Can you work these out from the drawing? Everything is in mm from the part's minimum corner. A direction names the side the tool comes from. Coordinates: 2 decimals unless noted, no trailing zeros. Order: outer loops, then holes, each group sorted by start corner. A loop starts at its lowest first (then second) coordinate and runs counter-clockwise, first axis right, second up. Notation, with made-up numbers: (18, 27.5) -> (49, 27.5) arc R4 ccw to (49, 32.5) -> close; hole circle Ø7 at (32.25, 32). An arc over 180 degrees is marked (long way). Return JSON: item names as keys, results as strings. Group by question number.
1) If I drill on probe 1 along Y at (x, z) = (9.5, 11); probe 2 along Z at (x, y) = (10, 6), over which ranges is the centre line in solid material (lowest first)? Write a range as from..to.
2) If we section it at B-B, the plane x = 5.5: Please give me the cut outline in (y, z), then the cut area to 3 significant figures.
3) If we section it at D-D, the plane x = 9: Please give me the cut outline in (y, z).
4) For pin 1 (4.5 mm diameter, centred on y = 10, z = 7.5, fed in from +X); pin 2 (6 mm diameter, centred on x = 10, z = 7.5, fed in from +Y); pin 3 (6 mm diameter, centred on y = 9.5, z = 9, fed in from +X), each with a flat end and sliding along its axis, tell me the tip position at first contact or that it passes through.
5) If we section it at C-C, the plane z = 13.25: Please give me the cut outline in (x, y), then the cut area to 3 significant figures.
6) If we section it at A-A, the plane z = 7.5: Please give me the cut outline in (x, y), then the cut area to 3 significant figures.
7) For the marked faces 4, 5 and 6, which set-ups out of +Z, -Z, +X, -X, +Y, -Y let a thin tool reach every point of the face, with its end or its side?
8) Thinking about a two-plate mould opening in Z: for the marked faces 1, 2 and 3, which applies, +Z half, -Z half, draft (parallel to the pull), parting line (faces both ways), or undercut?
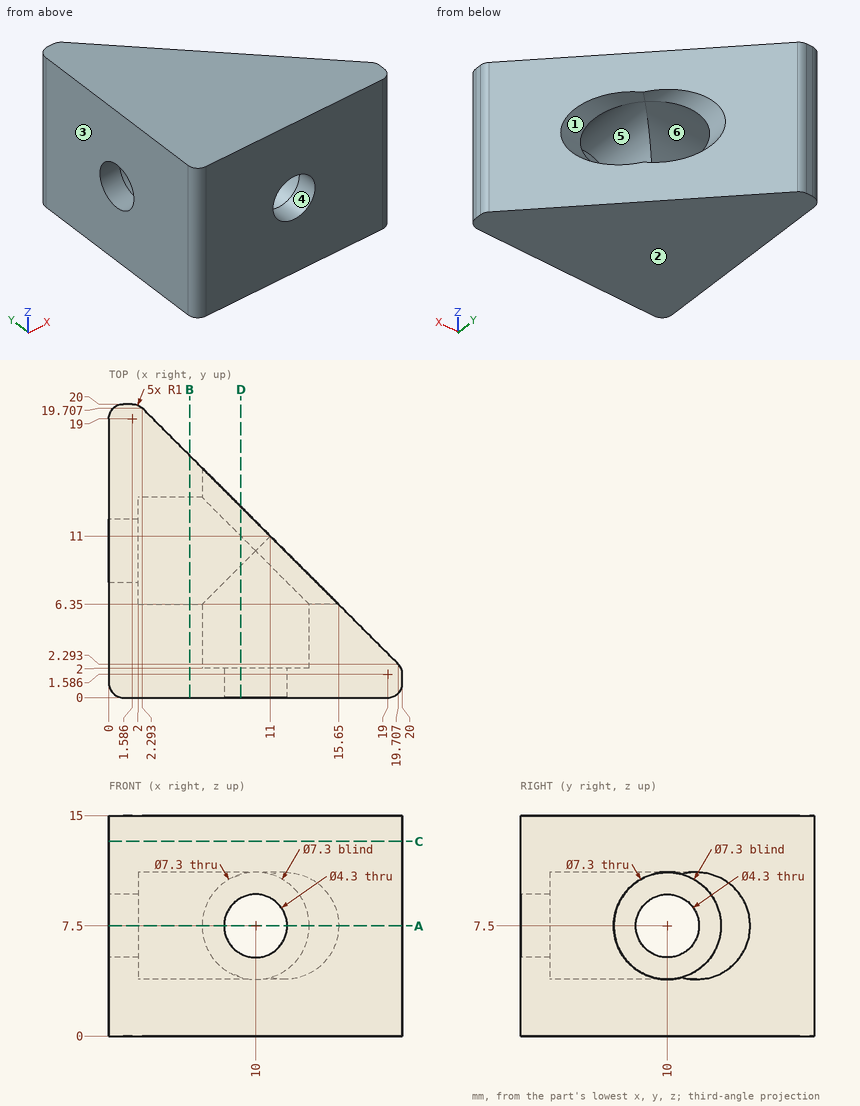
Result sheet:
{
 "1": {"probe 1": "y = 0..2", "probe 2": "z = 0..3.85, 11.15..15"},
 "2": {"outline": "(0, 0) -> (16.5, 0) -> (16.5, 15) -> (0, 15) -> close; hole circle Ø7.3 at (10, 7.5)", "area": "206 mm2"},
 "3": {"outline": "(0, 0) -> (13, 0) -> (13, 3.99) -> (11, 3.99) arc R3.65 cw to (9, 3.99) -> (2, 3.99) -> (2, 5.6) -> (0, 5.6) -> close; (0, 9.4) -> (2, 9.4) -> (2, 11.01) -> (9, 11.01) arc R3.65 cw to (11, 11.01) -> (13, 11.01) -> (13, 15) -> (0, 15) -> close"},
 "4": {"pin 1": "stops at x = 2", "pin 2": "stops at y = 2", "pin 3": "stops at x = 15.5"},
 "5": {"outline": "(0, 1) arc R1 ccw to (1, 0) -> (19, 0) arc R1 ccw to (20, 1) -> (20, 1.59) arc R1 ccw to (19.71, 2.29) -> (2.29, 19.71) arc R1 ccw to (1.59, 20) -> (1, 20) arc R1 ccw to (0, 19) -> close", "area": "237 mm2"},
 "6": {"outline": "(0, 1) arc R1 ccw to (1, 0) -> (7.85, 0) -> (7.85, 2) -> (6.35, 2) -> (6.35, 6.35) -> (2, 6.35) -> (2, 7.85) -> (0, 7.85) -> close; (0, 12.15) -> (2, 12.15) -> (2, 13.65) -> (6.35, 13.65) -> (6.35, 15.65) -> (2.29, 19.71) arc R1 ccw to (1.59, 20) -> (1, 20) arc R1 ccw to (0, 19) -> close; (12.15, 0) -> (19, 0) arc R1 ccw to (20, 1) -> (20, 1.59) arc R1 ccw to (19.71, 2.29) -> (15.65, 6.35) -> (13.65, 6.35) -> (13.65, 2) -> (12.15, 2) -> close", "area": "113 mm2"},
 "7": {"face 4": "+Y, -Y", "face 5": "+Y", "face 6": "+X"},
 "8": {"face 1": "undercut", "face 2": "-Z half", "face 3": "draft"}
}
